```python
from build123d import *

# Parameters (mm, degrees)
F0_R     = 22
F1_DEPTH = 3
F2_R     = 19.5
F3_DEPTH = 3
F4_R     = 4
F5_DEPTH = 6.001


with BuildPart() as f1:
    # F0 (on Top) → F1 (new body)
    with BuildSketch(Plane.XY):
        Circle(F0_R)
    extrude(amount=F1_DEPTH)

    # F2 (on face) → F3 (join)
    with BuildSketch(Plane.XY.offset(3)):
        Circle(F2_R)
    extrude(amount=F3_DEPTH)

    # F4 (on face) → F5 (cut, through all)
    with BuildSketch(Plane.XY.offset(6)):
        Circle(F4_R)
    extrude(amount=-F5_DEPTH, mode=Mode.SUBTRACT)


solid = f1.part
```
Geometry check sheet. Reference: the model listing, model coordinates, mm. Round coordinates to 2 decimals unless told otherwise and drop trailing zeros. Loops run counter-clockwise (first coordinate to the right, second up) from the corner with the lowest first, then second, coordinate; pieces in that order, holes last. Notation, with made-up numbers: (-26, 83.25) - (26, 83.25) arc R21 cw to (26, 100.25) - close; hole circle Ø3 at (79, 83.25). An arc over 180 degrees is marked (long way). Write item = value, one per line. Start each with the question number.
1. Section check C-C on z = 1.65. Enter the section's corners in (x, y), then the cut area to 3 significant figures.
2. Section check D-D on y = 5.5. Enter the section's corners in (x, z).
3. Mould release check, pull along Y, two halves, no side actions. Record for faces 1 (the face through (-0.867, -3.905, 3.042)), 2 (the face through (-2.539, 19.334, 4.479)), 3 (the face through (-13, -15, 3)): released by +Y, released by -Y, zero draft, split by the parting line, or undercut.
4. Depth check by flat-ended pin: pin 1 (2 mm diameter, centred on x = -9, z = 3, fed in from +Y); pin 2 (1 mm diameter, centred on y = 16.5, z = 1, fed in from -X); pin 3 (3 mm diameter, centred on x = 0.5, z = 3.5, fed in from +Y). Enter the tip coordinate at first touch or a pass-through.
5. Section check A-A on y = 0. Enter the section's corners in (x, z).
6. Thickness scan on line 1 (Y direction, x = 0, z = 2.7); line 2 (Y direction, x = 0, z = 4.05); line 3 (X direction, y = 3, z = 4.15). Record the ranges inside material, lowest first.
Working result:
q1.outline = circle Ø44 at (0, 0); hole circle Ø8 at (0, 0)
q1.area = 1,470 mm^2
q2.outline = (-21.3, 0) - (21.3, 0) - (21.3, 3) - (18.71, 3) - (18.71, 6) - (-18.71, 6) - (-18.71, 3) - (-21.3, 3) - close
q3.face_1 = undercut
q3.face_2 = split by the parting line
q3.face_3 = zero draft
q4.pin_1 = 20.49
q4.pin_2 = -15.1
q4.pin_3 = 22
q5.outline = (-22, 0) - (-4, 0) - (-4, 6) - (-19.5, 6) - (-19.5, 3) - (-22, 3) - close; (4, 0) - (22, 0) - (22, 3) - (19.5, 3) - (19.5, 6) - (4, 6) - close
q6.line_1 = -22 to -4, 4 to 22
q6.line_2 = -19.5 to -4, 4 to 19.5
q6.line_3 = -19.27 to -2.65, 2.65 to 19.27
